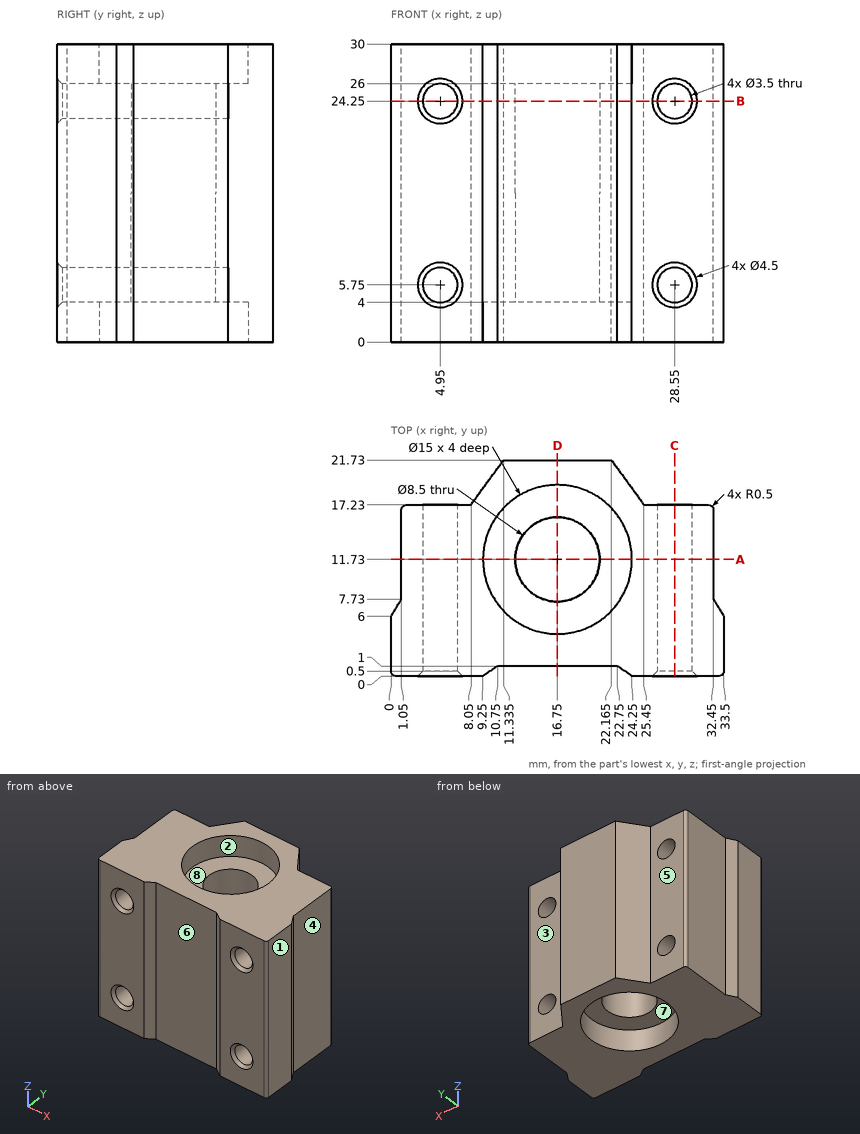
Input: dimensioned drawing with shaded views. Units: mm. Origin: part minimum x, y, z. A direction names the side the tool comes from. Round coordinates to 2 decimals unless told otherwise and drop trailing zeros. Loops run counter-clockwise (first coordinate to the right, second up) from the corner with the lowest first, then second, coordinate; pieces in that order, holes last. Notation, with made-up numbers: (75, -27) -> (122, -27) arc R22 ccw to (122, -14) -> close; hole circle Ø3 at (-39, -36). An arc over 180 degrees is marked (long way). Answer as a JSON object with one key per item and string values. Group by question number.
Q1. Mould query, pull axis Y, two halves, no side actions, for the marked faces 1, 2 and 3. Classes: pulls with the +Y half, pulls with the -Y half, needs draft (parallel to the pull), parting line crosses it, or undercut.
Q2. Section query A-A (y = 11.73). Output: boundary loops of the cut face in (x, z).
Q3. Contact query for flat-ended pins moving along their axis: P1, Ø4, axis at y = 12.5, z = 12, coming from the -X side; P2, Ø11, axis at x = 16.75, y = 11.73, coming from the +Z side; P3, Ø8, axis at x = 11, y = 12.5, coming from the -Z side; P4, Ø7, axis at x = 4.5, z = 10.5, coming from the +Y side. Output: stop coordinate, or through.
Q4. Access query for the marked faces 4, 5, 6, 7 and 8. Directions: +Z, -Z, +X, -X, +Y, -Y. A direction counts if a zero-diameter tool reaches every point of the face in a straight line with its end or side. Return the directions, or none.
Q5. Section query C-C (x = 28.55). Output: boundary loops of the cut face in (y, z).
Q6. Ray query, line 1 (Z direction, x = 28.55, y = 10.25); line 2 (Y direction, x = 16.5, z = 11.25); line 3 (Z direction, x = 6.5, y = 14.25). Return the intervals inside material, ascending. Write a range as from..to.
Q7. Section query D-D (x = 16.75). Output: boundary loops of the cut face in (y, z).
Q8. Section query B-B (z = 24.25). State how many separate pieces and enclosed holes the cut face has, plus the area to 3 significant figures.
Completed:
{
 "1": {"face 1": "needs draft", "face 2": "undercut", "face 3": "pulls with the +Y half"},
 "2": {"outline": "(1.05, 0) -> (9.25, 0) -> (9.25, 4) -> (12.5, 4) -> (12.5, 26) -> (9.25, 26) -> (9.25, 30) -> (1.05, 30) -> close; (21, 4) -> (24.25, 4) -> (24.25, 0) -> (32.45, 0) -> (32.45, 30) -> (24.25, 30) -> (24.25, 26) -> (21, 26) -> close; hole circle Ø3.5 at (4.95, 5.75); hole circle Ø3.5 at (4.95, 24.25); hole circle Ø3.5 at (28.55, 5.75); hole circle Ø3.5 at (28.55, 24.25)"},
 "3": {"P1": "x = 1.05", "P2": "z = 26", "P3": "z = 0", "P4": "y = 17.23"},
 "4": {"face 4": "+Z, -Z, +X, +Y", "face 5": "+Z, -Z, -X, +Y", "face 6": "+Z, -Z, -Y", "face 7": "-Z", "face 8": "+Z"},
 "5": {"outline": "(0, 0) -> (17.23, 0) -> (17.23, 4) -> (0.5, 4) -> (0, 3.5) -> close; (0, 8) -> (0.5, 7.5) -> (17.23, 7.5) -> (17.23, 22.5) -> (0.5, 22.5) -> (0, 22) -> close; (0, 26.5) -> (0.5, 26) -> (17.23, 26) -> (17.23, 30) -> (0, 30) -> close"},
 "6": {"line 1": "0..4, 7.5..22.5, 26..30", "line 2": "1..7.49, 15.97..21.73", "line 3": "0..4.94, 6.56..23.44, 25.06..30"},
 "7": {"outline": "(1, 0) -> (4.23, 0) -> (4.23, 4) -> (7.48, 4) -> (7.48, 26) -> (4.23, 26) -> (4.23, 30) -> (1, 30) -> close; (15.98, 4) -> (19.23, 4) -> (19.23, 0) -> (21.73, 0) -> (21.73, 30) -> (19.23, 30) -> (19.23, 26) -> (15.98, 26) -> close"},
 "8": {"separate pieces": "3", "enclosed holes": "1", "area": "427 mm²"}
}
